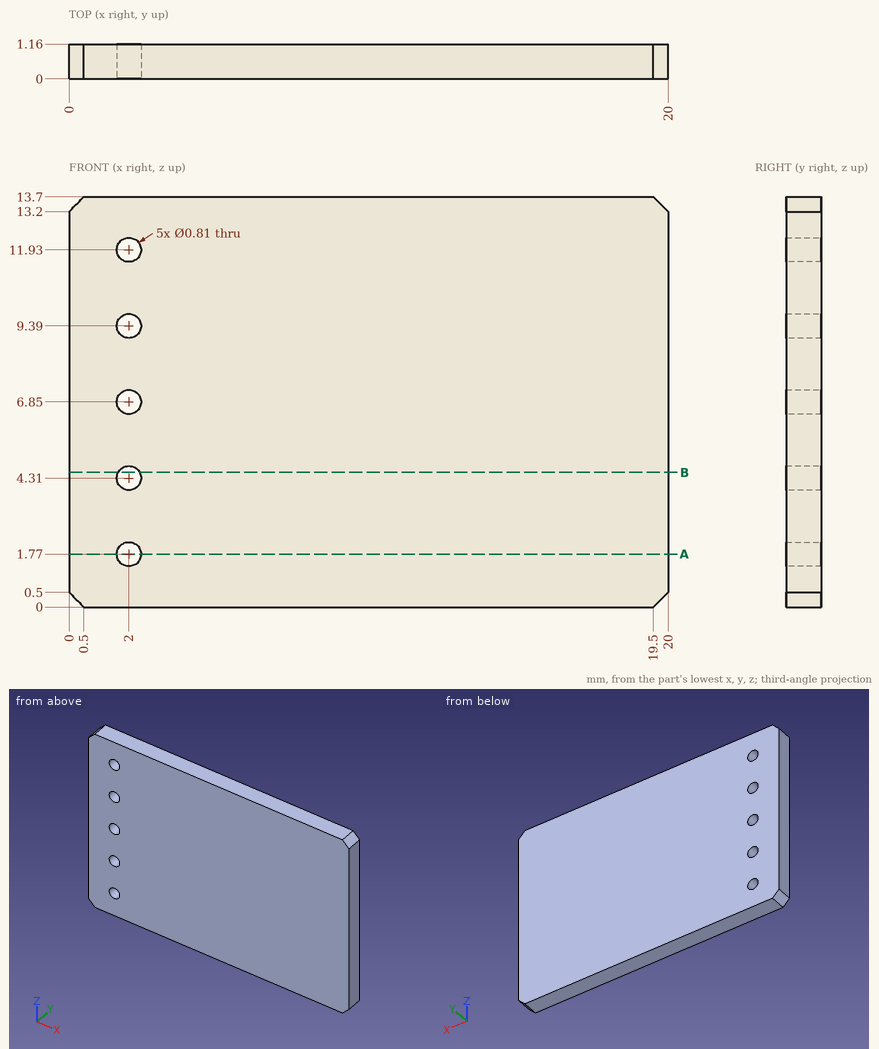
Source: three-view drawing plus pictorial views. Frame: mm from the lowest corner of the part. Coordinates: 2 decimals unless noted, no trailing zeros. Order: outer loops, then holes, each group sorted by start corner. A loop starts at its lowest first (then second) coordinate and runs counter-clockwise, first axis right, second up. Notation, with made-up numbers: M -2.5,38 L 1.5,38 A22 cw 1.5,53 Z; hole C -20,-15.75 d11. An arc over 180 degrees is marked long. Answer in a Markdown table with one row per item.
(1) Section query B-B, the plane z = 4.5. Output: boundary loops of the cut face in (x, y), plus the area to 3 significant figures.
Numbers:
| item | result |
|---|---|
| outline | M 0,0 L 1.64,0 L 1.64,1.16 L 0,1.16 Z; M 2.36,0 L 20,0 L 20,1.16 L 2.36,1.16 Z |
| area | 22.4 mm^2 |
(2) Material intervals for line 1 (X direction, y = 0.75, z = 1.77) (3 decimals), sorted ascending. Write a range as [from, to].
Numbers:
| item | result |
|---|---|
| line 1 | x = [0, 1.595], [2.405, 20] |
(3) Section query A-A, the plane z = 1.77. Output: boundary loops of the cut face in (x, y) (3 decimals), plus the area to 3 significant figures.
Numbers:
| item | result |
|---|---|
| outline | M 0,0 L 1.595,0 L 1.595,1.16 L 0,1.16 Z; M 2.405,0 L 20,0 L 20,1.16 L 2.405,1.16 Z |
| area | 22.3 mm^2 |
